Geometry check sheet. Reference: the model listing, model coordinates, mm. Face numbers are marked on the shaded views. A direction names the side the tool comes from. Give positions to 0.01 mm unless a question says otherwise; leave off trailing zeros. Write each loop counter-clockwise with the first axis right and the second up, starting at its lowest first coordinate (ties: lowest second). Pieces come first, ordered by that corner, then holes. Notation, with made-up numbers: (20.5, 27) - (41.5, 27) arc R15 cw to (41.5, 53) - close; hole circle Ø4 at (58, -36). An arc over 180 degrees is marked (long way). Write item = value, one per line. Start each with the question number.
(1) Thickness scan on L1, parallel to Y at x = 3, z = -23; L2, parallel to X at y = 3.2, z = -23; L3, parallel to Z at x = 8, y = 0. Record the ranges inside material, lowest first.
(2) Section check C-C, the plane z = -23. Give the number of separate pieces and of enclosed holes in the cut face, plus the area to 3 significant figures.
(3) Draft check along Y on the marked faces 1, 2 and 3. Enter one of: pulls with the +Y half, pulls with the -Y half, needs draft (parallel to the pull), parting line crosses it, or undercut.
(4) Depth check by flat-ended pin: pin 1 Ø1 at (y, z) = (-4.5, 5.5) entering from +X; pin 2 Ø6 at (x, z) = (7.5, -24) entering from +Y; pin 3 Ø16 at (y, z) = (0, 0) entering from -X. Enter the tip coordinate at first touch or a pass-through.
(5) Section check A-A, the plane z = 0. Enter the section's corners in (x, y), plus the area to 3 significant figures.
(6) Section check B-B, the plane x = 3.75. Enter the section's corners in (y, z).
(7) Access from +Z, -Z, +X, -X, +Y, -Y to the whole of each face (thin tool, end or side, straight path). Record for the marked faces 4, 5, 6 and 7.
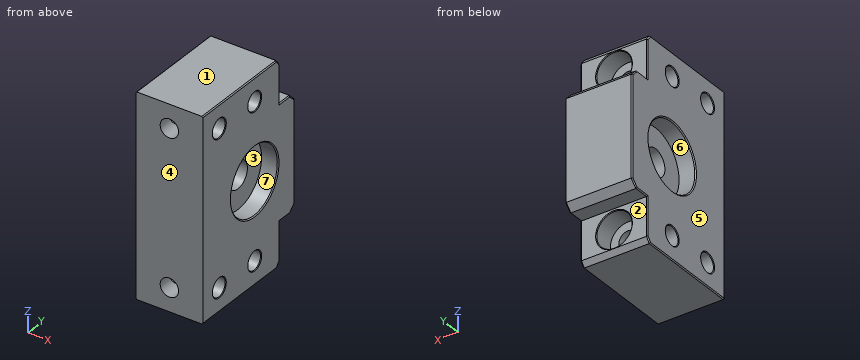
```python
from build123d import *

# Parameters (mm, degrees)
SKETCH1_R                      = 4
SKETCH1_R_2                    = 2.75
BOSS_EXTRUDE1_DEPTH            = 20
SKETCH2_R                      = 10
CUT_EXTRUDE1_DEPTH             = 5
CUT_EXTRUDE2_START             = -5
SKETCH3_R                      = 10
CUT_EXTRUDE2_DEPTH             = 5
CHAMFER2_SIZE                  = 0.2
CHAMFER3_SIZE                  = 0.2
CHAMFER4_SIZE                  = 0.2
CUT_EXTRUDE4_REACH             = 55.113
SKETCH4_R                      = 2.75
CUT_EXTRUDE4_DIRECTION_2_DEPTH = 54.1130869
SKETCH5_R                      = 5.3
CUT_EXTRUDE6_DEPTH             = 6
SKETCH6_R                      = 5.3
CUT_EXTRUDE7_DEPTH             = 6
CHAMFER6_SIZE                  = 0.2
CHAMFER7_SIZE                  = 0.2
CHAMFER11_SIZE                 = 0.3
CHAMFER12_SIZE                 = 0.3


# Some blends are built 0.0001 mm under size
with BuildPart() as part:
    # Sketch1 → Boss-Extrude1 (new body)
    with BuildSketch(Plane(origin=(0, 0, 0), x_dir=(0, 0, -1), z_dir=(1, 0, 0))):
        Polygon((-30, -22), (30, -22), (30, 9.32807156), (28.5, 10.5), (17, 10.5), (17, 15), (15, 17), (-15, 17), (-17, 15), (-17, 10.5), (-28.5, 10.499728155), (-30, 9.327742612), align=None)
        Circle(SKETCH1_R, mode=Mode.SUBTRACT)
        with Locations((-23, 0)):
            Circle(SKETCH1_R_2, mode=Mode.SUBTRACT)
        with Locations((23, 0)):
            Circle(SKETCH1_R_2, mode=Mode.SUBTRACT)
        with Locations((23, -15)):
            Circle(SKETCH1_R_2, mode=Mode.SUBTRACT)
        with Locations((-23, -15)):
            Circle(SKETCH1_R_2, mode=Mode.SUBTRACT)
    extrude(amount=BOSS_EXTRUDE1_DEPTH)

    # Sketch2 → Cut-Extrude1 (cut)
    with BuildSketch(Plane.ZY):
        Circle(SKETCH2_R)
    extrude(amount=-CUT_EXTRUDE1_DEPTH, mode=Mode.SUBTRACT)

    # Sketch3 → Cut-Extrude2 (cut)
    with BuildSketch(Plane(origin=(20, 0, 0), x_dir=(0, 0, -1), z_dir=(1, 0, 0)).offset(CUT_EXTRUDE2_START)):
        with Locations(Location((0, 0, 0), (0, 0, 180))):
            Circle(SKETCH3_R)
    extrude(amount=CUT_EXTRUDE2_DEPTH, mode=Mode.SUBTRACT)

    # Chamfer2
    chamfer2_edges = [part.edges().sort_by_distance(p)[0] for p in [
        (0, 0, -20.25),
    ]]
    chamfer(chamfer2_edges, length=CHAMFER2_SIZE)

    # Chamfer3
    chamfer3_edges = [part.edges().sort_by_distance(p)[0] for p in [
        (0, 0, 25.75),
        (0, -15, -20.25),
        (0, -15, 25.75),
    ]]
    chamfer(chamfer3_edges, length=CHAMFER3_SIZE)

    # Chamfer4
    chamfer4_edges = [part.edges().sort_by_distance(p)[0] for p in [
        (20, 0, -20.25),
        (20, 0, 25.75),
        (20, -15, -20.25),
        (20, -15, 25.75),
    ]]
    chamfer(chamfer4_edges, length=CHAMFER4_SIZE)

    # Cut-Extrude4: up to this face of the body (flat: up to its plane)
    cut_extrude4_end = Plane(part.part.faces().sort_by_distance((10, 10.5, -22.75))[0])
    # Sketch4 → Cut-Extrude4 (cut, up to the picked face)
    with BuildSketch(Plane.XZ.offset(22), mode=Mode.PRIVATE) as cut_extrude4_sk1:
        with Locations(Location((10, 23, 0), (0, 0, 270))):
            Circle(SKETCH4_R)
    cut_extrude4_tool1 = split(extrude(cut_extrude4_sk1.sketch, amount=-CUT_EXTRUDE4_REACH, mode=Mode.PRIVATE), bisect_by=cut_extrude4_end, keep=Keep.BOTH, mode=Mode.PRIVATE)
    # Sketch4 → Cut-Extrude4 (cut, up to the picked face)
    with BuildSketch(Plane.XZ.offset(22), mode=Mode.PRIVATE) as cut_extrude4_sk2:
        with Locations(Location((10, -23, 0), (0, 0, 270))):
            Circle(SKETCH4_R)
    cut_extrude4_tool2 = split(extrude(cut_extrude4_sk2.sketch, amount=-CUT_EXTRUDE4_REACH, mode=Mode.PRIVATE), bisect_by=cut_extrude4_end, keep=Keep.BOTH, mode=Mode.PRIVATE)
    add(cut_extrude4_tool1.solids().sort_by(Axis((10, -22, 23), (0, 1, 0)))[0], mode=Mode.SUBTRACT)
    add(cut_extrude4_tool2.solids().sort_by(Axis((10, -22, -23), (0, 1, 0)))[0], mode=Mode.SUBTRACT)

    # Sketch4 → Cut-Extrude4 direction 2 (cut)
    with BuildSketch(Plane.XZ.offset(22)):
        with Locations(Location((10, 23, 0), (0, 0, 270))):
            Circle(SKETCH4_R)
        with Locations(Location((10, -23, 0), (0, 0, 270))):
            Circle(SKETCH4_R)
    extrude(amount=CUT_EXTRUDE4_DIRECTION_2_DEPTH, mode=Mode.SUBTRACT)

    # Sketch5 → Cut-Extrude6 (cut)
    with BuildSketch(Plane(origin=(0, 10.5, 0), x_dir=(1, 0, 0), z_dir=(0, 1, 0))):
        with Locations(Location((10, 23, 0), (0, 0, 270))):
            Circle(SKETCH5_R)
    extrude(amount=-CUT_EXTRUDE6_DEPTH, mode=Mode.SUBTRACT)

    # Sketch6 → Cut-Extrude7 (cut)
    with BuildSketch(Plane(origin=(0, 10.500401852, 0.000248216), x_dir=(1, 0, 0), z_dir=(0, 0.9999999997206055, 2.3638723279467724e-05))):
        with Locations(Location((10, -23.000354574, 0), (0, 0, 270))):
            Circle(SKETCH6_R)
    extrude(amount=-CUT_EXTRUDE7_DEPTH, mode=Mode.SUBTRACT)

    # Chamfer6
    # the kernel refuses this chamfer: 0.2 mm, written as the material it takes off along each edge
    with BuildSketch(Plane(origin=(10, 10.499858153, 23.000602784), x_dir=(0, -2.363872327936284e-05, 0.9999999997206054), z_dir=(-1, 0, 0))) as chamfer6_piece_1:
        Polygon((5.3 + CHAMFER6_SIZE, 0), (5.3, -CHAMFER6_SIZE), (5.3, 0), align=None)
    revolve(axis=Axis((10, 10.499858153, 23.000602784), (0, 0.9999999997206055, 2.3638723279467724e-05)), mode=Mode.SUBTRACT)

    # Chamfer7
    chamfer7_edges = [part.edges().sort_by_distance(p)[0] for p in [
        (10, 10.5, -28.3),
    ]]
    chamfer(chamfer7_edges, length=CHAMFER7_SIZE - 0.0001)  # a hair under: the kernel refuses the full size

    # Chamfer11
    chamfer11_edges = [part.edges().sort_by_distance(p)[0] for p in [
        (20, -6.336128694, 30),
        (20, -6.33596422, -30),
        (20, 9.91403578, -29.25),
        (20, 10.5, -22.75),
        (20, 12.75, -17),
        (20, 16, -16),
        (20, 17, 0),
        (20, 16, 16),
        (20, 12.75, 17),
        (20, 10.499864077, 22.75),
        (20, 0, -10),
        (20, 9.913735383, 29.25),
    ]]
    chamfer(chamfer11_edges, length=CHAMFER11_SIZE)

    # Chamfer12
    chamfer12_edges = [part.edges().sort_by_distance(p)[0] for p in [
        (0, 12.75, 17),
        (0, 16, 16),
        (0, 17, 0),
        (0, 16, -16),
        (0, 12.75, -17),
        (0, 10.5, -22.75),
        (0, 9.91403578, -29.25),
        (0, -6.33596422, -30),
        (0, -6.336128694, 30),
        (0, 9.913735383, 29.25),
        (0, 10.499864077, 22.75),
        (0, 0, -10),
    ]]
    chamfer(chamfer12_edges, length=CHAMFER12_SIZE)


solid = part.part
```
Model answer:
q1.L1 = -22 to -17.75, -12.25 to -2.75, 2.75 to 10.5
q1.L2 = 0 to 7.25, 12.75 to 20
q1.L3 = -30 to -25.75, -20.25 to -4, 4 to 20.25, 25.75 to 30
q2.separate_pieces = 6
q2.enclosed_holes = 0
q2.area = 281 mm²
q3.face_1 = needs draft
q3.face_2 = pulls with the +Y half
q3.face_3 = undercut
q4.pin_1 = 15
q4.pin_2 = 10.5
q4.pin_3 = 5
q5.outline = (0, -22) - (20, -22) - (20, -10.3) - (19.7, -10) - (15, -10) - (15, -4) - (5, -4) - (5, -10) - (0.3, -10) - (0, -10.3) - close; (0, 10.3) - (0.3, 10) - (5, 10) - (5, 4) - (15, 4) - (15, 10) - (19.7, 10) - (20, 10.3) - (20, 16.7) - (19.7, 17) - (0.3, 17) - (0, 16.7) - close
q5.area = 500 mm²
q6.outline = (-22, -30) - (9.33, -30) - (10.5, -28.5) - (10.5, -17) - (15, -17) - (17, -15) - (17, 15) - (15, 17) - (10.5, 17) - (10.5, 28.5) - (9.33, 30) - (-22, 30) - close; hole circle Ø5.5 at (-15, -23); hole circle Ø5.5 at (-15, 23); hole circle Ø20 at (0, 0); hole circle Ø5.5 at (0, -23); hole circle Ø5.5 at (0, 23)
q7.face_4 = +Z, -Z, +X, -X, -Y
q7.face_5 = +Z, -Z, -X, +Y, -Y
q7.face_6 = -X
q7.face_7 = +X
